Input: dimensioned drawing with shaded views. Units: mm. Origin: part minimum x, y, z. A direction names the side the tool comes from. Give positions to 0.01 mm unless a question says otherwise; leave off trailing zeros. Loops run counter-clockwise (first coordinate to the right, second up) from the corner with the lowest first, then second, coordinate; pieces in that order, holes last. Notation, with made-up numbers: (11, -2) -> (28, -2) arc R14 cw to (28, 21) -> close; hole circle Ø1 at (11, -11.5). An arc over 180 degrees is marked (long way). Answer in a Markdown table with one row per item. Add a question column.
1) Access query for the marked faces 1, 2 and 3. Directions: +Z, -Z, +X, -X, +Y, -Y. A direction counts if a zero-diameter tool reaches every point of the face in a straight line with its end or side. Return the directions, or none.
2) Section query C-C (z = 19.25). Return the cut outline in (x, y).
3) Section query B-B (x = 32.5). Return the cut outline in (y, z), plus the area to 3 significant figures.
4) First-contact query: P1, Ø3, axis at y = 18, z = 14, coming from the -X side; P2, Ø11, axis at x = 38, z = 17.5, coming from the -Y side; P3, Ø3, axis at y = 5, z = 21, coming from the +X side. Flat tips, straight axial feed; report the tip coordinate or a pass-through.
5) Line query: line 1 (Y direction, x = 32.5, z = 22); line 2 (X direction, y = 17, z = 18.75); line 3 (Z direction, x = 6, y = 18.25). Output: solid intervals per line, ascending. Write a range as from..to.
6) Section query A-A (y = 10.5). Return the cut outline in (x, z).
7) Section query D-D (y = 25.75). Return the cut outline in (x, z), plus the area to 3 significant figures.
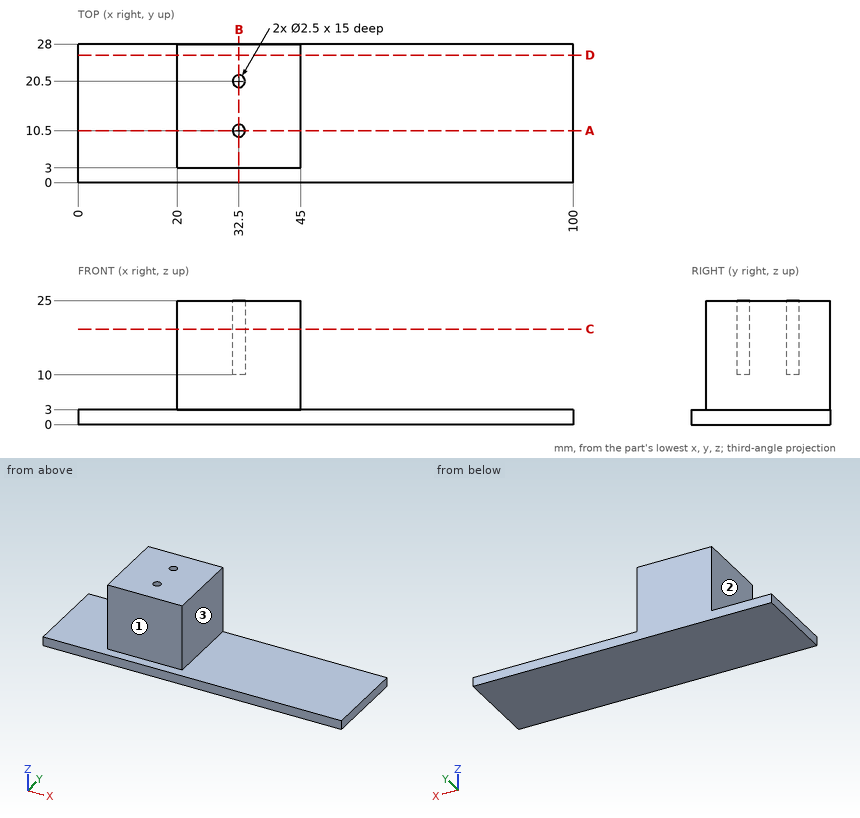
Evaluation:
| question | item | result |
|---|---|---|
| 1 | face 1 | +Z, +X, -X, -Y |
| 1 | face 2 | +Z, -X, +Y, -Y |
| 1 | face 3 | +Z, +X, +Y, -Y |
| 2 | outline | (20, 3) -> (45, 3) -> (45, 28) -> (20, 28) -> close; hole circle Ø2.5 at (32.5, 10.5); hole circle Ø2.5 at (32.5, 20.5) |
| 3 | outline | (0, 0) -> (28, 0) -> (28, 25) -> (21.75, 25) -> (21.75, 10) -> (19.25, 10) -> (19.25, 25) -> (11.75, 25) -> (11.75, 10) -> (9.25, 10) -> (9.25, 25) -> (3, 25) -> (3, 3) -> (0, 3) -> close |
| 3 | area | 559 mm² |
| 4 | P1 | x = 20 |
| 4 | P2 | y = 3 |
| 4 | P3 | x = 45 |
| 5 | line 1 | 3..9.25, 11.75..19.25, 21.75..28 |
| 5 | line 2 | 20..45 |
| 5 | line 3 | 0..3 |
| 6 | outline | (0, 0) -> (100, 0) -> (100, 3) -> (45, 3) -> (45, 25) -> (33.75, 25) -> (33.75, 10) -> (31.25, 10) -> (31.25, 25) -> (20, 25) -> (20, 3) -> (0, 3) -> close |
| 7 | outline | (0, 0) -> (100, 0) -> (100, 3) -> (45, 3) -> (45, 25) -> (20, 25) -> (20, 3) -> (0, 3) -> close |
| 7 | area | 850 mm² |
